CAD build for the part. Positions are in the model's coordinates, mm. A direction names the side the tool comes from. Round coordinates to 2 decimals unless told otherwise and drop trailing zeros. Loops run counter-clockwise (first coordinate to the right, second up) from the corner with the lowest first, then second, coordinate; pieces in that order, holes last.
```python
from build123d import *

# Parameters (mm, degrees)
F0_W     = 228.6
F0_H     = 25.4
F1_DEPTH = 63.5
F3_DEPTH = 50.8
F5_DEPTH = 139.7


with BuildPart() as f1:
    # F0 (on Right) → F1 (new body, symmetric)
    with BuildSketch(Plane.YZ):
        with Locations((114.3, 12.7)):
            Rectangle(F0_W, F0_H)
    extrude(amount=F1_DEPTH, both=True)

    # F2 (on Right) → F3 (join, symmetric)
    with BuildSketch(Plane.YZ):
        with BuildLine():
            Line((127, 6.35), (127, 44.803873))
            ThreePointArc((127, 44.803873), (76.2, 177.8), (25.4, 44.803873))
            Line((25.4, 44.803873), (25.4, 6.35))
            Line((25.4, 6.35), (127, 6.35))
        make_face()
    extrude(amount=F3_DEPTH, both=True)

    # F4 (on Front) → F5 (join)
    with BuildSketch(Plane.XZ):
        with BuildLine():
            Line((-50.8, 184.15), (-50.8, 171.45))
            Line((-50.8, 171.45), (50.8, 171.45))
            Line((50.8, 171.45), (50.8, 184.15))
            ThreePointArc((50.8, 184.15), (43.360512, 202.110512), (25.4, 209.55))
            Line((25.4, 209.55), (18.872138, 209.55))
            Line((18.872138, 209.55), (18.872138, 206.375))
            Line((18.872138, 206.375), (16.527231, 206.375))
            Line((16.527231, 206.375), (16.527231, 209.55))
            Line((16.527231, 209.55), (6.172138, 209.55))
            Line((6.172138, 209.55), (6.172138, 206.375))
            Line((6.172138, 206.375), (3.827231, 206.375))
            Line((3.827231, 206.375), (3.827231, 209.55))
            Line((3.827231, 209.55), (-6.527862, 209.55))
            Line((-6.527862, 209.55), (-6.527862, 206.375))
            Line((-6.527862, 206.375), (-8.872769, 206.375))
            Line((-8.872769, 206.375), (-8.872769, 209.55))
            Line((-8.872769, 209.55), (-19.227862, 209.55))
            Line((-19.227862, 209.55), (-19.227862, 206.375))
            Line((-19.227862, 206.375), (-21.572769, 206.375))
            Line((-21.572769, 206.375), (-21.572769, 209.55))
            Line((-21.572769, 209.55), (-25.4, 209.55))
            ThreePointArc((-25.4, 209.55), (-43.360512, 202.110512), (-50.8, 184.15))
        make_face()
    extrude(amount=-F5_DEPTH)


solid = f1.part
```
Item 1: Probe line 1 (Z direction, x = -8, y = 16) (3 decimals); line 2 (Z direction, x = -56.5, y = 63.5); line 3 (X direction, y = 62.5, z = 107). List the from-to ranges inside material, lowest first.
Answers follow:
line 1: z = 0 to 25.4, 54.884 to 148.316, 171.45 to 206.375
line 2: z = 0 to 25.4
line 3: x = -50.8 to 50.8
Item 2: 3-axis set-ups, long thin cutter, end or side, ignore diameter. For faces 1 (the flat face through (-1, 23, 171.45)), 2 (the flat face through (-50.8, 75, 106)), 3 (the flat face through (-1, 139.7, 191)): which of +Z, -Z, +X, -X, +Y, -Y reach the whole face in a straight line?
Answers follow:
face 1: +X, -X, -Y
face 2: +Z, -X, +Y, -Y
face 3: +Z, +X, -X, +Y
Item 3: Cut at C-C, the plane x = -2. Give the cut face in (y, z).
Answers follow:
outline: (0, 0) - (228.6, 0) - (228.6, 25.4) - (127, 25.4) - (127, 44.8) arc R76.2 ccw to (106.65, 171.45) - (139.7, 171.45) - (139.7, 209.55) - (0, 209.55) - (0, 171.45) - (45.75, 171.45) arc R76.2 ccw to (25.4, 44.8) - (25.4, 25.4) - (0, 25.4) - close
Item 4: Two-plate mould, pull along Z, no slides. Class faces 4 (the flat face through (1, 138, 25.4)), 5 (the flat face through (1, 113, 0)), 6 (the flat face through (-1, 69, 209.55)), 7 (the flat face through (-1, 123, 171.45)): released by +Z, released by -Z, zero draft, split by the parting line, or undercut.
Answers follow:
face 4: undercut
face 5: released by -Z
face 6: released by +Z
face 7: undercut
Item 5: Cut at D-D, the plane z = 32. Give the cut face in (x, y).
Answers follow:
outline: (-50.8, 25.4) - (50.8, 25.4) - (50.8, 127) - (-50.8, 127) - close
Item 6: Cut at B-B, the plane y = 51.5. Give the cut face in (x, z) (3 decimals), plus the area to 3 significant figures.
Answers follow:
outline: (-63.5, 0) - (63.5, 0) - (63.5, 25.4) - (50.8, 25.4) - (50.8, 184.15) arc R25.4 ccw to (25.4, 209.55) - (18.872, 209.55) - (18.872, 206.375) - (16.527, 206.375) - (16.527, 209.55) - (6.172, 209.55) - (6.172, 206.375) - (3.827, 206.375) - (3.827, 209.55) - (-6.528, 209.55) - (-6.528, 206.375) - (-8.873, 206.375) - (-8.873, 209.55) - (-19.228, 209.55) - (-19.228, 206.375) - (-21.573, 206.375) - (-21.573, 209.55) - (-25.4, 209.55) arc R25.4 ccw to (-50.8, 184.15) - (-50.8, 25.4) - (-63.5, 25.4) - close
area: 21,600 mm2
Item 7: Flat gauge pins, fed straight in: P1, Ø2.5, axis at y = 51.5, z = 207.5, coming from the -X side; P2, Ø1, axis at x = 15, z = 28, coming from the -Y side; P3, Ø3, axis at y = 64.5, z = 121.5, coming from the +X side. Where does each tip first touch, or does it go through?
Answers follow:
P1: stops at x = -37.92
P2: stops at y = 25.4
P3: stops at x = 50.8
